```python
from build123d import *

# Parameters (mm, degrees)
SKETCH1_W                                  = 500
SKETCH1_H                                  = 400
BOSS_EXTRUDE1_DEPTH                        = 4.5
SKETCH2_W                                  = 4.4
SKETCH2_H                                  = 200
CUT_EXTRUDE1_DEPTH                         = 4.5
SKETCH5_W                                  = 50
SKETCH5_H                                  = 4.4
CUT_EXTRUDE2_DEPTH                         = 4.5
MIRROR5_AT_THE_SECOND_PLANE_COPY_1_SKETC_W = 50
MIRROR5_AT_THE_SECOND_PLANE_COPY_1_SKETC_H = 4.4
MIRROR5_AT_THE_SECOND_PLANE_COPY_1_DEPTH   = 4.5


with BuildPart() as part:
    # Sketch1 → Boss-Extrude1 (new body)
    with BuildSketch(Plane(origin=(0, 0, 0), x_dir=(1, 0, 0), z_dir=(0, 1, 0))):
        Rectangle(SKETCH1_W, SKETCH1_H)
    extrude(amount=BOSS_EXTRUDE1_DEPTH)

    # Sketch2 → Cut-Extrude1 (cut)
    with BuildSketch(Plane(origin=(0, 4.5, 0), x_dir=(1, 0, 0), z_dir=(0, 1, 0))):
        with Locations((-152.2, 0)):
            Rectangle(SKETCH2_W, SKETCH2_H)
    cut_extrude1 = extrude(amount=-CUT_EXTRUDE1_DEPTH, mode=Mode.SUBTRACT)

    # Mirror2: Cut-Extrude1 across plane
    add(cut_extrude1.mirror(Plane(origin=(0, 0, 0), x_dir=(0, 0, 1), z_dir=(1, 0, 0))), mode=Mode.SUBTRACT)

    # Sketch5 → Cut-Extrude2 (cut)
    with BuildSketch(Plane(origin=(0, 4.5, 0), x_dir=(1, 0, 0), z_dir=(0, 1, 0))):
        with Locations((-199.9, 147.8)):
            Rectangle(SKETCH5_W, SKETCH5_H)
    cut_extrude2 = extrude(amount=-CUT_EXTRUDE2_DEPTH, mode=Mode.SUBTRACT)

    # Mirror5: Cut-Extrude2 across plane
    add(cut_extrude2.mirror(Plane.XY), mode=Mode.SUBTRACT)

    # Mirror5 at the second plane: Cut-Extrude2 across plane
    add(cut_extrude2.mirror(Plane(origin=(0, 0, 0), x_dir=(0, 0, 1), z_dir=(1, 0, 0))), mode=Mode.SUBTRACT)

    # Mirror5 at the second plane copy 1 sketc → Mirror5 at the second plane copy 1 (cut)
    with BuildSketch(Plane(origin=(0, 4.5, 0), x_dir=(-1, 0, 0), z_dir=(0, 1, 0))):
        with Locations((-199.9, 147.8)):
            Rectangle(MIRROR5_AT_THE_SECOND_PLANE_COPY_1_SKETC_W, MIRROR5_AT_THE_SECOND_PLANE_COPY_1_SKETC_H)
    extrude(amount=-MIRROR5_AT_THE_SECOND_PLANE_COPY_1_DEPTH, mode=Mode.SUBTRACT)


solid = part.part
```
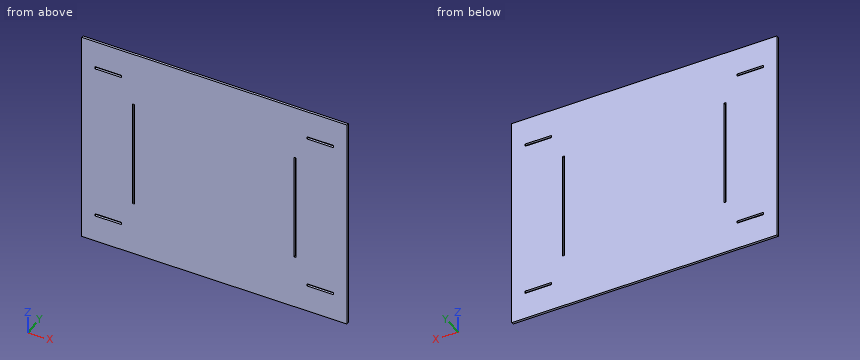
Here's how the part is built. I have some questions about the finished solid (model axes, mm). Give positions to 0.01 mm unless a question says otherwise; leave off trailing zeros. Order: outer loops, then holes, each group sorted by start corner. A loop starts at its lowest first (then second) coordinate and runs counter-clockwise, first axis right, second up. Notation, with made-up numbers: (49.5, 16.25) - (87.5, 16.25) arc R33 ccw to (87.5, 50.25) - close; hole circle Ø2 at (70, 35). An arc over 180 degrees is marked (long way). Answer as a JSON object with one key per item and string values. Group by question number.
Item 1: Please list where these lines run through material, in increasing order: probe 1 along Z at (x, y) = (222, 2.3); probe 2 along X at (y, z) = (0.8, 99.5).
Item 2: If we section it at A-A on z = 5: Please give me the cut outline in (x, y).
Item 3: If we section it at B-B on x = -181: Please give me the cut outline in (y, z), and give its area (3 significant figures).
Result set:
{
 "1": {"probe 1": "-200 to -150, -145.6 to 145.6, 150 to 200", "probe 2": "-250 to -154.4, -150 to 150, 154.4 to 250"},
 "2": {"outline": "(-250, 0) - (-154.4, 0) - (-154.4, 4.5) - (-250, 4.5) - close; (-150, 0) - (150, 0) - (150, 4.5) - (-150, 4.5) - close; (154.4, 0) - (250, 0) - (250, 4.5) - (154.4, 4.5) - close"},
 "3": {"outline": "(0, -200) - (4.5, -200) - (4.5, -150) - (0, -150) - close; (0, -145.6) - (4.5, -145.6) - (4.5, 145.6) - (0, 145.6) - close; (0, 150) - (4.5, 150) - (4.5, 200) - (0, 200) - close", "area": "1,760 mm²"}
}
